Could you check a few things on this model? Use its own coordinates, in mm. Face numbers are marked on the shaded views. Give positions to 0.01 mm unless a question says otherwise; leave off trailing zeros. Order: outer loops, then holes, each group sorted by start corner. A loop starts at its lowest first (then second) coordinate and runs counter-clockwise, first axis right, second up.
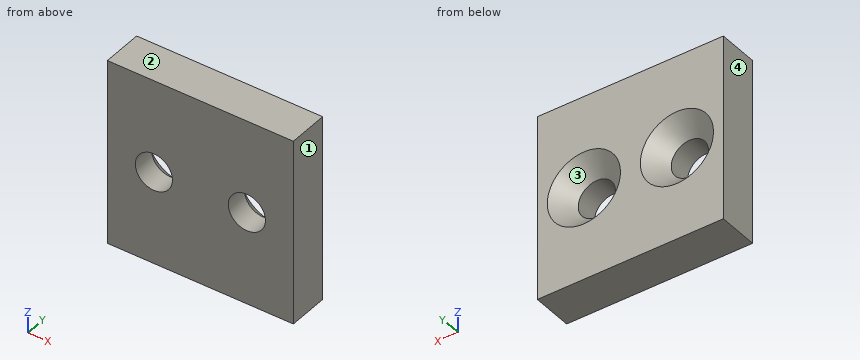
from build123d import *

# Parameters (mm, degrees)
SKETCH1_W           = 32
SKETCH1_H           = 32
BOSS_EXTRUDE1_DEPTH = 7
HOLE1_D             = 6.4
HOLE1_DEPTH         = 7
HOLE1_CSINK_D       = 12.6
HOLE1_CSINK_ANGLE   = 90


with BuildPart() as part:
    # Sketch1 → Boss-Extrude1 (new body)
    with BuildSketch(Plane(origin=(0, 0, 0), x_dir=(1, 0, 0), z_dir=(0, 1, 0))):
        Rectangle(SKETCH1_W, SKETCH1_H)
    extrude(amount=BOSS_EXTRUDE1_DEPTH)

    # Hole1
    with Locations(Plane(origin=(0, 7, 0), x_dir=(1, 0, 0), z_dir=(0, 1, 0))):
        with Locations((8, 0), (-8, 0)):
            CounterSinkHole(HOLE1_D / 2, HOLE1_CSINK_D / 2, depth=HOLE1_DEPTH, counter_sink_angle=HOLE1_CSINK_ANGLE)


solid = part.part
Item 1: For pin 1 (8.5 mm diameter, centred on x = 8, z = 0, fed in from +Y); pin 2 (7.5 mm diameter, centred on x = -8, z = 0, fed in from +Y), each with a flat end and sliding along its axis, tell me the tip position at first contact or that it passes through.
Findings:
pin 1: stops at y = 4.95
pin 2: stops at y = 4.45
Item 2: Imagine slicing it at B-B on y = 6. List the corners of the cut face in (x, z) for me.
Findings:
outline: (-16, -16) - (16, -16) - (16, 16) - (-16, 16) - close; hole circle Ø10.6 at (-8, 0); hole circle Ø10.6 at (8, 0)
Item 3: Please list where these lines run through material, in increasing order: line 1 along Z through (x, y) = (8, 3.15); line 2 along Z through (x, y) = (7.5, 6.25); line 3 along Y through (x, z) = (11, -3.5).
Findings:
line 1: z = -16 to -3.2, 3.2 to 16
line 2: z = -16 to -5.53, 5.53 to 16
line 3: y = 0 to 5.31
Item 4: Imagine slicing it at C-C on z = 0. List the corners of the cut face in (x, y) for me.
Findings:
outline: (-16, 0) - (-11.2, 0) - (-11.2, 3.9) - (-14.3, 7) - (-16, 7) - close; (-4.8, 0) - (4.8, 0) - (4.8, 3.9) - (1.7, 7) - (-1.7, 7) - (-4.8, 3.9) - close; (11.2, 0) - (16, 0) - (16, 7) - (14.3, 7) - (11.2, 3.9) - close
Item 5: We'd pull the mould along X, two halves only. Please class the marked faces 1, 2, 3 and 4: +X half, -X half, draft (parallel to the pull), parting line (faces both ways), or undercut.
Findings:
face 1: +X half
face 2: draft
face 3: undercut
face 4: -X half
Item 6: Imagine slicing it at A-A on x = 8. List the corners of the cut face in (y, z) for me, then the cut area to 3 significant figures.
Findings:
outline: (0, -16) - (7, -16) - (7, -6.3) - (3.9, -3.2) - (0, -3.2) - close; (0, 3.2) - (3.9, 3.2) - (7, 6.3) - (7, 16) - (0, 16) - close
area: 170 mm2
Item 7: Imagine slicing it at D-D on y = 2.75. List the corners of the cut face in (x, z) for me.
Findings:
outline: (-16, -16) - (16, -16) - (16, 16) - (-16, 16) - close; hole circle Ø6.4 at (-8, 0); hole circle Ø6.4 at (8, 0)
